from build123d import *

# Parameters (mm, degrees)
SKETCH1_W           = 203.2
SKETCH1_H           = 101.6
SKETCH1_R           = 1.5
SKETCH1_W_2         = 173.2
SKETCH1_H_2         = 71.6
SKETCH1_W_3         = 25.4
BOSS_EXTRUDE1_DEPTH = 3.175
SKETCH2_R           = 2
SKETCH2_R_2         = 4
CUT_EXTRUDE1_DEPTH  = 3.175
SKETCH3_R           = 1.5
CUT_EXTRUDE2_DEPTH  = 10
SKETCH4_R           = 3.175
CUT_EXTRUDE3_DEPTH  = 10
SKETCH5_R           = 1.5
CUT_EXTRUDE4_DEPTH  = 10


with BuildPart() as part:
    # Sketch1 → Boss-Extrude1 (new body)
    # profile 1 of 2: a face of its own
    with BuildSketch(Plane(origin=(0, 0, 0), x_dir=(1, 0, 0), z_dir=(0, 1, 0))):
        with Locations((101.6, 50.8)):
            Rectangle(SKETCH1_W, SKETCH1_H)
        with Locations(Location((6.35, 95.25, 0), (0, 0, 270))):
            Circle(SKETCH1_R, mode=Mode.SUBTRACT)
        with Locations(Location((6.35, 88.9, 0), (0, 0, 270))):
            Circle(SKETCH1_R, mode=Mode.SUBTRACT)
        with Locations(Location((6.35, 6.35, 0), (0, 0, 270))):
            Circle(SKETCH1_R, mode=Mode.SUBTRACT)
        with Locations(Location((6.35, 12.7, 0), (0, 0, 270))):
            Circle(SKETCH1_R, mode=Mode.SUBTRACT)
        with Locations(Location((196.85, 95.25, 0), (0, 0, 270))):
            Circle(SKETCH1_R, mode=Mode.SUBTRACT)
        with Locations(Location((196.85, 88.9, 0), (0, 0, 270))):
            Circle(SKETCH1_R, mode=Mode.SUBTRACT)
        with Locations(Location((196.85, 12.7, 0), (0, 0, 270))):
            Circle(SKETCH1_R, mode=Mode.SUBTRACT)
        with Locations(Location((196.85, 6.35, 0), (0, 0, 270))):
            Circle(SKETCH1_R, mode=Mode.SUBTRACT)
        with Locations((101.6, 50.8)):
            Rectangle(SKETCH1_W_2, SKETCH1_H_2, mode=Mode.SUBTRACT)
    # profile 2 of 2: a face of its own
    with BuildSketch(Plane(origin=(0, 0, 0), x_dir=(1, 0, 0), z_dir=(0, 1, 0))):
        with Locations((99.246196593, 152.4)):
            Rectangle(SKETCH1_W_3, SKETCH1_H)
    extrude(amount=BOSS_EXTRUDE1_DEPTH)

    # Sketch2 → Cut-Extrude1 (cut)
    with BuildSketch(Plane(origin=(0, 3.175, 0), x_dir=(1, 0, 0), z_dir=(0, 1, 0))):
        with Locations(Location((91.246196593, 109.6, 0), (0, 0, 270))):
            Circle(SKETCH2_R)
        with Locations(Location((107.246196593, 109.6, 0), (0, 0, 270))):
            Circle(SKETCH2_R)
        with Locations(Location((91.246196593, 93.6, 0), (0, 0, 270))):
            Circle(SKETCH2_R)
        with Locations(Location((107.246196593, 93.6, 0), (0, 0, 270))):
            Circle(SKETCH2_R)
        with Locations(Location((99.246196593, 101.6, 0), (0, 0, 270))):
            Circle(SKETCH2_R_2)
    extrude(amount=-CUT_EXTRUDE1_DEPTH, mode=Mode.SUBTRACT)

    # Sketch3 → Cut-Extrude2 (cut)
    with BuildSketch(Plane(origin=(0, 3.175, 0), x_dir=(1, 0, 0), z_dir=(0, 1, 0))):
        with Locations(Location((178.2, 94.1, 0), (0, 0, 270))):
            Circle(SKETCH3_R)
        with Locations(Location((25, 94.1, 0), (0, 0, 270))):
            Circle(SKETCH3_R)
        with Locations(Location((76.546196593, 94.1, 0), (0, 0, 270))):
            Circle(SKETCH3_R)
        with Locations(Location((121.946196593, 94.1, 0), (0, 0, 270))):
            Circle(SKETCH3_R)
        with Locations(Location((178.2, 7.5, 0), (0, 0, 270))):
            Circle(SKETCH3_R)
        with Locations(Location((25, 7.5, 0), (0, 0, 270))):
            Circle(SKETCH3_R)
        with Locations(Location((195.7, 76.6, 0), (0, 0, 270))):
            Circle(SKETCH3_R)
        with Locations(Location((195.7, 25, 0), (0, 0, 270))):
            Circle(SKETCH3_R)
        with Locations(Location((7.5, 76.6, 0), (0, 0, 270))):
            Circle(SKETCH3_R)
        with Locations(Location((7.5, 25, 0), (0, 0, 270))):
            Circle(SKETCH3_R)
    extrude(amount=-CUT_EXTRUDE2_DEPTH, mode=Mode.SUBTRACT)

    # Sketch4 → Cut-Extrude3 (cut)
    with BuildSketch(Plane(origin=(0, 3.175, 0), x_dir=(1, 0, 0), z_dir=(0, 1, 0))):
        with Locations(Location((99.246196593, 190.5, 0), (0, 0, 270))):
            Circle(SKETCH4_R)
    extrude(amount=-CUT_EXTRUDE3_DEPTH, mode=Mode.SUBTRACT)

    # Sketch5 → Cut-Extrude4 (cut)
    with BuildSketch(Plane(origin=(0, 3.175, 0), x_dir=(1, 0, 0), z_dir=(0, 1, 0))):
        with Locations(Location((99.246196593, 177.8, 0), (0, 0, 270))):
            Circle(SKETCH5_R)
        with Locations(Location((99.246196593, 127, 0), (0, 0, 270))):
            Circle(SKETCH5_R)
    extrude(amount=-CUT_EXTRUDE4_DEPTH, mode=Mode.SUBTRACT)


solid = part.part
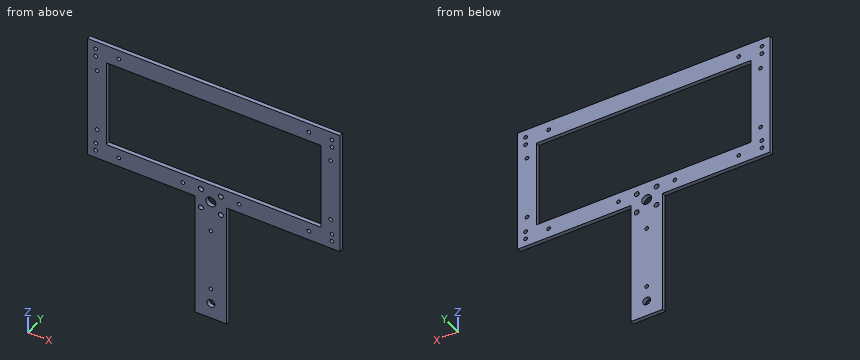
Can you work these out from the model? Positions are in its coordinate system, mm. Give positions to 0.01 mm unless a question says otherwise; leave off trailing zeros. Write each loop counter-clockwise with the first axis right and the second up, starting at its lowest first coordinate (ties: lowest second). Pieces come first, ordered by that corner, then holes. Notation, with made-up numbers: M 89,-22.5 L 120,-22.5 A6 ccw 120,-11.5 Z; hole C 0,22 d9. An arc over 180 degrees is marked long. Answer in a Markdown table with one row per item. Add a question column.
Item 1: Imagine slicing it at D-D, the plane x = 191. Write out the boundary of the cut face in (y, z) (3 decimals).
Item 2: For pin 1 Ø3.5 at (x, z) = (7.5, -25) entering from +Y (3 decimals); pin 2 Ø1.6 at (x, y) = (60.5, 1.5) entering from -Z, each with a flat end and sliding along its axis, tell me the tip position at first contact or that it passes through.
Item 3: Imagine slicing it at A-A, the plane x = 32.5. Write out the boundary of the cut face in (y, z) (3 decimals), plus the area to 4 significant figures.
Item 4: Imagine slicing it at B-B, the plane z = -17.5. Write out the boundary of the cut face in (x, y) (3 decimals).
Item 5: Please list where these lines run through material, in increasing order: L1, parallel to Z at x = 178.2, y = 1; L2, parallel to Z at x = 99, y = 3.05; L3, parallel to X at y = 0.8, z = -38.
Item 6: Imagine slicing it at C-C, the plane z = -182. Write out the boundary of the cut face in (x, y) (3 decimals), plus the area to 3 significant figures.
Evaluation:
| question | item | result |
|---|---|---|
| 1 | outline | M 0,-101.6 L 3.175,-101.6 L 3.175,0 L 0,0 Z |
| 2 | pin 1 | stops at y = 3.175 |
| 2 | pin 2 | stops at z = -101.6 |
| 3 | outline | M 0,-101.6 L 3.175,-101.6 L 3.175,-86.6 L 0,-86.6 Z; M 0,-15 L 3.175,-15 L 3.175,0 L 0,0 Z |
| 3 | area | 95.25 mm² |
| 4 | outline | M 0,0 L 15,0 L 15,3.175 L 0,3.175 Z; M 188.2,0 L 203.2,0 L 203.2,3.175 L 188.2,3.175 Z |
| 5 | L1 | z = -101.6 to -95.6, -92.6 to -86.6, -15 to -9, -6 to 0 |
| 5 | L2 | z = -203.2 to -193.67, -187.33 to -179.28, -176.32 to -128.48, -125.52 to -105.59, -97.61 to -86.6, -15 to 0 |
| 5 | L3 | x = 0 to 15, 188.2 to 203.2 |
| 6 | outline | M 86.546,0 L 111.946,0 L 111.946,3.175 L 86.546,3.175 Z |
| 6 | area | 80.6 mm² |
